```python
from build123d import *

# Parameters (mm, degrees)
F0_W     = 76.2
F0_H     = 54.356
F1_DEPTH = 50.8
F2_W     = 40.435703
F2_H     = 38.392941
F3_DEPTH = 50.8


with BuildPart() as f1:
    # F0 (on Top) → F1 (new body)
    with BuildSketch(Plane.XY):
        Rectangle(F0_W, F0_H)
    extrude(amount=F1_DEPTH)

    # F2 (on face) → F3 (cut)
    with BuildSketch(Plane.YZ.offset(38.1)):
        with Locations((0.132361, 25.30353)):
            Rectangle(F2_W, F2_H)
    extrude(amount=-F3_DEPTH, mode=Mode.SUBTRACT)


solid = f1.part
```
Here's how the part is built. I have some questions about the finished solid (model axes, mm). A direction names the side the tool comes from. Give positions to 0.01 mm unless a question says otherwise; leave off trailing zeros. Write each loop counter-clockwise with the first axis right and the second up, starting at its lowest first coordinate (ties: lowest second). Pieces come first, ordered by that corner, then holes.
(1) Imagine slicing it at A-A, the plane x = -10. Write out the boundary of the cut face in (y, z).
Output values:
outline: (-27.18, 0) - (27.18, 0) - (27.18, 50.8) - (-27.18, 50.8) - close; hole (-20.09, 6.11) - (20.35, 6.11) - (20.35, 44.5) - (-20.09, 44.5) - close
(2) Will this pin go through, and if not, where does the flat tip stop? pin 1 (6 mm diameter, centred on y = -3, z = 37, fed in from +X).
Output values:
pin 1: stops at x = -12.7
(3) Imagine slicing it at C-C, the plane y = -17. Write out the boundary of the cut face in (x, z).
Output values:
outline: (-38.1, 0) - (38.1, 0) - (38.1, 6.11) - (-12.7, 6.11) - (-12.7, 44.5) - (38.1, 44.5) - (38.1, 50.8) - (-38.1, 50.8) - close
(4) Imagine slicing it at B-B, the plane z = 28. Write out the boundary of the cut face in (x, y).
Output values:
outline: (-38.1, -27.18) - (38.1, -27.18) - (38.1, -20.09) - (-12.7, -20.09) - (-12.7, 20.35) - (38.1, 20.35) - (38.1, 27.18) - (-38.1, 27.18) - close
(5) Thinking about a two-plate mould opening in Z: for faces 1 (the face through (13, 0, 6.107)), 2 (the face through (-1, 0, 50.8)), 3 (the face through (-1, 27.178, 25)), which applies, pulls with the +Z half, pulls with the -Z half, needs draft (parallel to the pull), parting line crosses it, or undercut?
Output values:
face 1: undercut
face 2: pulls with the +Z half
face 3: needs draft
(6) If I drill on L1, parallel to Y at x = 17, z = 15.5; L2, parallel to Z at x = 2.5, y = 17; L3, parallel to X at y = -10, z = 38, over which ranges is the centre line in solid material (lowest first)?
Output values:
L1: y = -27.18 to -20.09, 20.35 to 27.18
L2: z = 0 to 6.11, 44.5 to 50.8
L3: x = -38.1 to -12.7
(7) On a 3-axis mill with a long thin cutter (end or side, diameter ignored), from which of +Z, -Z, +X, -X, +Y, -Y can I reach the whole of each face in a straight line? I mean faces 4 (the face through (38.1, 0, 48)), 5 (the face through (-12.7, 0, 26)). Say none if no direction works.
Output values:
face 4: +Z, -Z, +X, +Y, -Y
face 5: +X
